```python
from build123d import *

# Parameters (mm, degrees)
SKIZZE1_W                       = 97
SKIZZE1_H                       = 41.280710538
AUFSATZ_LINEAR_AUSTRAGEN1_DEPTH = 1.2
AUFSATZ_LINEAR_AUSTRAGEN2_DEPTH = 50
SKIZZE3_W                       = 23.3
SKIZZE3_H                       = 19.6
SKIZZE3_W_2                     = 16.4
SKIZZE3_H_2                     = 14.8
AUFSATZ_LINEAR_AUSTRAGEN3_DEPTH = 3
SKIZZE3_2_W                     = 16.4
SKIZZE3_2_H                     = 14.8
SCHNITT_LINEAR_AUSTRAGEN1_DEPTH = 117.203171482
SKIZZE5_W                       = 97
SKIZZE5_H                       = 41.280710538
AUFSATZ_LINEAR_AUSTRAGEN4_DEPTH = 1.2
SKIZZE7_W                       = 4.6
SKIZZE7_H                       = 4.6
SKIZZE7_R                       = 1.425
AUFSATZ_LINEAR_AUSTRAGEN5_DEPTH = 12
SKIZZE8_R                       = 1.75
SCHNITT_LINEAR_AUSTRAGEN3_DEPTH = 12
SKIZZE9_W                       = 6
SKIZZE9_H                       = 10
SCHNITT_LINEAR_AUSTRAGEN4_DEPTH = 12
SKIZZE10_W                      = 4.6
SKIZZE10_H                      = 4.6
AUFSATZ_LINEAR_AUSTRAGEN6_DEPTH = 0.6
FASE1_SIZE                      = 4.6


with BuildPart() as part:
    # Skizze1 → Aufsatz-Linear austragen1 (new body)
    with BuildSketch(Plane.XY):
        with Locations((48.5, 20.640355269)):
            Rectangle(SKIZZE1_W, SKIZZE1_H)
    extrude(amount=AUFSATZ_LINEAR_AUSTRAGEN1_DEPTH)

    # Skizze2 → Aufsatz-Linear austragen2 (add)
    with BuildSketch(Plane.XY.offset(1.2)):
        Polygon((0, 41.280710538), (0, 0), (48.5, 0), (97, 0), (97, 41.280710538), (95.8, 41.280710538), (95.8, 0.6), (1.2, 0.6), (1.2, 41.280710538), align=None)
    extrude(amount=AUFSATZ_LINEAR_AUSTRAGEN2_DEPTH)

    # Skizze3 → Aufsatz-Linear austragen3 (add)
    with BuildSketch(Plane(origin=(1.2, 0, 0), x_dir=(0, 0, -1), z_dir=(1, 0, 0))):
        with Locations((-39.55, 10.4)):
            Rectangle(SKIZZE3_W, SKIZZE3_H)
        with Locations((-39.1, 9.8)):
            Rectangle(SKIZZE3_W_2, SKIZZE3_H_2, mode=Mode.SUBTRACT)
    extrude(amount=AUFSATZ_LINEAR_AUSTRAGEN3_DEPTH)

    # Skizze3<2> → Schnitt-Linear austragen1 (cut, through all)
    with BuildSketch(Plane(origin=(1.2, 0, 0), x_dir=(0, 0, -1), z_dir=(1, 0, 0))):
        with Locations((-39.1, 9.8)):
            Rectangle(SKIZZE3_2_W, SKIZZE3_2_H)
    extrude(amount=-SCHNITT_LINEAR_AUSTRAGEN1_DEPTH, mode=Mode.SUBTRACT)

    # Skizze5 → Aufsatz-Linear austragen4 (add)
    with BuildSketch(Plane.XY.offset(51.2)):
        with Locations((48.5, 20.640355269)):
            Rectangle(SKIZZE5_W, SKIZZE5_H)
    extrude(amount=AUFSATZ_LINEAR_AUSTRAGEN4_DEPTH)

    # Skizze7 → Aufsatz-Linear austragen5 (add)
    # profile 1 of 4: a face of its own
    with BuildSketch(Plane(origin=(0, 41.280710538, 0), x_dir=(1, 0, 0), z_dir=(0, 1, 0))):
        with Locations((3.5, -3.5)):
            Rectangle(SKIZZE7_W, SKIZZE7_H)
        with Locations(Location((2.7, -2.7, 0), (0, 0, 270))):
            Circle(SKIZZE7_R, mode=Mode.SUBTRACT)
    # profile 2 of 4: a face of its own
    with BuildSketch(Plane(origin=(0, 41.280710538, 0), x_dir=(1, 0, 0), z_dir=(0, 1, 0))):
        with Locations((93.5, -3.5)):
            Rectangle(SKIZZE7_W, SKIZZE7_H)
        with Locations(Location((94.3, -2.7, 0), (0, 0, 90))):
            Circle(SKIZZE7_R, mode=Mode.SUBTRACT)
    # profile 3 of 4: a face of its own
    with BuildSketch(Plane(origin=(0, 41.280710538, 0), x_dir=(1, 0, 0), z_dir=(0, 1, 0))):
        with Locations((93.5, -48.9)):
            Rectangle(SKIZZE7_W, SKIZZE7_H)
        with Locations(Location((94.3, -49.7, 0), (0, 0, 270))):
            Circle(SKIZZE7_R, mode=Mode.SUBTRACT)
    # profile 4 of 4: a face of its own
    with BuildSketch(Plane(origin=(0, 41.280710538, 0), x_dir=(1, 0, 0), z_dir=(0, 1, 0))):
        with Locations((3.5, -48.9)):
            Rectangle(SKIZZE7_W, SKIZZE7_H)
        with Locations(Location((2.7, -49.7, 0), (0, 0, 90))):
            Circle(SKIZZE7_R, mode=Mode.SUBTRACT)
    extrude(amount=-AUFSATZ_LINEAR_AUSTRAGEN5_DEPTH)

    # Skizze8 → Schnitt-Linear austragen3 (cut)
    with BuildSketch(Plane.XY.offset(1.2)):
        with Locations((11.25, 7.530710538)):
            Circle(SKIZZE8_R)
        with Locations((43.25, 7.530710538)):
            Circle(SKIZZE8_R)
        with Locations((53.75, 7.530710538)):
            Circle(SKIZZE8_R)
        with Locations((85.75, 7.530710538)):
            Circle(SKIZZE8_R)
    extrude(amount=-SCHNITT_LINEAR_AUSTRAGEN3_DEPTH, mode=Mode.SUBTRACT)

    # Skizze9 → Schnitt-Linear austragen4 (cut)
    with BuildSketch(Plane.ZY):
        with Locations((9.605096132, 7.910310386)):
            Rectangle(SKIZZE9_W, SKIZZE9_H)
    extrude(amount=-SCHNITT_LINEAR_AUSTRAGEN4_DEPTH, mode=Mode.SUBTRACT)

    # Skizze10 → Aufsatz-Linear austragen6 (add)
    with BuildSketch(Plane.XZ.offset(-29.280710538)):
        with Locations((3.5, 48.9)):
            Rectangle(SKIZZE10_W, SKIZZE10_H)
        with Locations((3.5, 3.5)):
            Rectangle(SKIZZE10_W, SKIZZE10_H)
        with Locations((93.5, 48.9)):
            Rectangle(SKIZZE10_W, SKIZZE10_H)
        with Locations((93.5, 3.5)):
            Rectangle(SKIZZE10_W, SKIZZE10_H)
    extrude(amount=AUFSATZ_LINEAR_AUSTRAGEN6_DEPTH)

    # Fase1
    fase1_edges = [part.edges().sort_by_distance(p)[0] for p in [
        (1.2, 28.680710538, 3.5),
        (3.5, 28.680710538, 1.2),
        (93.5, 28.680710538, 1.2),
        (95.8, 28.680710538, 3.5),
        (95.8, 28.680710538, 48.9),
        (93.5, 28.680710538, 51.2),
        (1.2, 28.680710538, 48.9),
        (3.5, 28.680710538, 51.2),
    ]]
    chamfer(fase1_edges, length=FASE1_SIZE - 0.0001)  # a hair under: the kernel refuses the full size


solid = part.part
```
Work out the finished part from the listing and answer in its coordinate system (mm). A direction names the side the tool comes from. Give positions to 0.01 mm unless a question says otherwise; leave off trailing zeros. Loops run counter-clockwise (first coordinate to the right, second up) from the corner with the lowest first, then second, coordinate; pieces in that order, holes last. Notation, with made-up numbers: (66, -22) -> (82, -22) arc R8 ccw to (82, -15) -> close; hole circle Ø7 at (65.5, 24). An arc over 180 degrees is marked (long way). One line per question, with ' | ' between items. Start each with the question number.
1) Determine the mould class of faces 1 (the face through (3, 35, 46.6)), 2 (the face through (48, 0, 26)), 3 (the face through (92.96, 25.84, 2.96)) for opening direction Y: +Y half, -Y half, draft (parallel to the pull), parting line (faces both ways), or undercut.
2) Section B-B, the plane x = 11.25 is taken. Determine the outline of the cut face in (y, z), then the cut area to 3 significant figures.
3) Section D-D, the plane y = 22 is taken. Determine the outline of the cut face in (x, z), then the cut area to 3 significant figures.
4) This flat-tipped pin is pushed along its axis until it touches: pin 1 (8 mm diameter, centred on x = 72, z = 43, fed in from +Y). Where does it stop, or does it pass through?
5) For faces 4 (the face through (93, 35, 5.8)), 5 (the face through (4.2, 10.5, 47.5)), 6 (the face through (2, 17.2, 39)), 7 (the face through (44.867, 6.86, 0.608)), determine the directions among +Z, -Z, +X, -X, +Y, -Y from which every point of the face is accessible in a straight line to the end or side of a thin tool.
6) Section C-C, the plane z = 10.5 is taken. Determine the outline of the cut face in (x, y).
7) Straight lines are drawn through the part: L1, parallel to X at y = 33, z = 49.7 (3 decimals); L2, parallel to Z at x = 94.3, y = 37 (3 decimals); L3, parallel to X at y = 39, z = 23.5. For each, find the intervals that lie inside material, in ascending order.
8) Section A-A, the plane y = 11.5 is taken. Determine the outline of the cut face in (x, z), then the cut area to 3 significant figures.
Resolved:
1) face 1: draft | face 2: -Y half | face 3: undercut
2) outline: (0, 0) -> (5.78, 0) -> (5.78, 1.2) -> (0.6, 1.2) -> (0.6, 51.2) -> (41.28, 51.2) -> (41.28, 52.4) -> (0, 52.4) -> close; (9.28, 0) -> (41.28, 0) -> (41.28, 1.2) -> (9.28, 1.2) -> close | area: 125 mm2
3) outline: (0, 0) -> (97, 0) -> (97, 52.4) -> (0, 52.4) -> close; hole (1.2, 1.2) -> (95.8, 1.2) -> (95.8, 51.2) -> (1.2, 51.2) -> close | area: 353 mm2
4) pin 1: y = 0.6
5) face 4: +Y | face 5: none | face 6: -X | face 7: -Z
6) outline: (0, 0) -> (97, 0) -> (97, 41.28) -> (95.8, 41.28) -> (95.8, 0.6) -> (1.2, 0.6) -> (1.2, 2.91) -> (0, 2.91) -> close; (0, 12.91) -> (1.2, 12.91) -> (1.2, 41.28) -> (0, 41.28) -> close
7) L1: 0 to 1.275, 4.125 to 5.8, 91.2 to 92.875, 95.725 to 97 | L2: 0 to 1.275, 4.125 to 5.8, 46.6 to 48.275, 51.125 to 52.4 | L3: 0 to 1.2, 95.8 to 97
8) outline: (0, 0) -> (97, 0) -> (97, 52.4) -> (0, 52.4) -> (0, 47.3) -> (4.2, 47.3) -> (4.2, 51.2) -> (95.8, 51.2) -> (95.8, 1.2) -> (1.2, 1.2) -> (1.2, 6.61) -> (0, 6.61) -> close; (0, 12.61) -> (1.2, 12.61) -> (1.2, 27.9) -> (4.2, 27.9) -> (4.2, 30.9) -> (0, 30.9) -> close | area: 347 mm2
